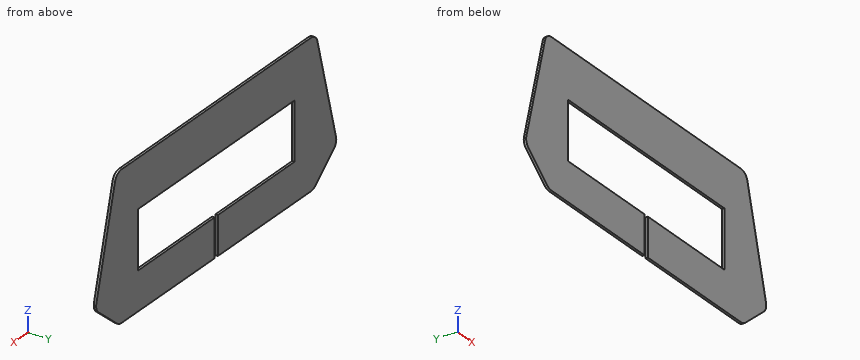
```python
from build123d import *

# Parameters (mm, degrees)
BASE_FLANGE1_DEPTH = 0.25


# Sheet-metal steps are written as plain solids
with BuildPart() as part:
    # Sketch1 → Base-Flange1 (new body)
    with BuildSketch(Plane(origin=(0, 0, 0), x_dir=(1, 0, 0), z_dir=(0, 1, 0))):
        with BuildLine():
            Line((-14.178620776, -8), (14.178620776, -8))
            ThreePointArc((14.178620776, -8), (14.789399734, -7.791801152), (15.145851741, -7.253898128))
            Line((15.145851741, -7.253898128), (17.939776994, 3.389626646))
            ThreePointArc((17.939776994, 3.389626646), (17.926022481, 3.944992277), (17.618005902, 4.407318956))
            Line((17.618005902, 4.407318956), (14.829510217, 6.763794182))
            ThreePointArc((14.829510217, 6.763794182), (14.527711383, 6.939093761), (14.184050345, 7))
            Line((14.184050345, 7), (0.25, 7))
            Line((0.25, 7), (0.25, 3))
            Line((0.25, 3), (11.7, 3))
            Line((11.7, 3), (11.7, -3))
            Line((11.7, -3), (-11.7, -3))
            Line((-11.7, -3), (-11.7, 3))
            Line((-11.7, 3), (-0.25, 3))
            Line((-0.25, 3), (-0.25, 7))
            Line((-0.25, 7), (-14.184050345, 7))
            ThreePointArc((-14.184050345, 7), (-14.527711383, 6.939093761), (-14.829510217, 6.763794182))
            Line((-14.829510217, 6.763794182), (-17.618005902, 4.407318956))
            ThreePointArc((-17.618005902, 4.407318956), (-17.926022481, 3.944992277), (-17.939776994, 3.389626646))
            Line((-17.939776994, 3.389626646), (-15.145851741, -7.253898128))
            ThreePointArc((-15.145851741, -7.253898128), (-14.789399734, -7.791801152), (-14.178620776, -8))
        make_face()
    extrude(amount=-BASE_FLANGE1_DEPTH)


solid = part.part
```
CAD build for the part. Positions are in the model's coordinates, mm. Coordinates: 2 decimals unless noted, no trailing zeros. Loops run counter-clockwise (first coordinate to the right, second up) from the corner with the lowest first, then second, coordinate; pieces in that order, holes last. Notation, with made-up numbers: (-25.5, 8) - (30.5, 8) arc R21 cw to (30.5, 32) - close; hole circle Ø9 at (-32, 86.5). An arc over 180 degrees is marked (long way). Return JSON: item names as keys, results as strings.
1. Band-saw the part on B-B (z = 0.75). Give the cut face in (x, y), and give its area (3 significant figures).
Result:
{"outline": "(-16.85, -0.25) - (-11.7, -0.25) - (-11.7, 0) - (-16.85, 0) - close; (11.7, -0.25) - (16.85, -0.25) - (16.85, 0) - (11.7, 0) - close", "area": "2.58 mm2"}
2. Drop a flat-ended pin along its axis: pin 1 (3 mm diameter, centred on x = -11, z = -0.5, fed in from -Y). Give the stop position or say it passes through.
Result:
{"pin 1": "stops at y = -0.25"}
3. Band-saw the part on D-D (z = 4.5). Give the cut face in (x, y).
Result:
{"outline": "(-15.87, -0.25) - (15.87, -0.25) - (15.87, 0) - (-15.87, 0) - close"}
4. Band-saw the part on C-C (y = -0.1). Give the cut face in (x, z).
Result:
{"outline": "(-17.94, -3.39) arc R1 ccw to (-17.62, -4.41) - (-14.83, -6.76) arc R1 ccw to (-14.18, -7) - (-0.25, -7) - (-0.25, -3) - (-11.7, -3) - (-11.7, 3) - (11.7, 3) - (11.7, -3) - (0.25, -3) - (0.25, -7) - (14.18, -7) arc R1 ccw to (14.83, -6.76) - (17.62, -4.41) arc R1 ccw to (17.94, -3.39) - (15.15, 7.25) arc R1 ccw to (14.18, 8) - (-14.18, 8) arc R1 ccw to (-15.15, 7.25) - close"}
5. Probe L1, parallel to Z at x = -6.5, y = -0.05; L2, parallel to X at y = -0.2, z = -4.75; L3, parallel to X at y = -0.15, z = 1.5. List the from-to ranges inside material, lowest first. Write a range as from..to.
Result:
{"L1": "z = -7..-3, 3..8", "L2": "x = -17.21..-0.25, 0.25..17.21", "L3": "x = -16.66..-11.7, 11.7..16.66"}
6. Band-saw the part on A-A (x = 7). Give the cut face in (y, z).
Result:
{"outline": "(-0.25, -7) - (0, -7) - (0, -3) - (-0.25, -3) - close; (-0.25, 3) - (0, 3) - (0, 8) - (-0.25, 8) - close"}
